Geometry: final body of the model. Coordinates: model frame, mm. A direction names the side the tool comes from. Give positions to 0.01 mm unless a question says otherwise; leave off trailing zeros. Write each loop counter-clockwise with the first axis right and the second up, starting at its lowest first coordinate (ties: lowest second). Pieces come first, ordered by that corner, then holes. Notation, with made-up numbers: (33, -34.75) -> (62, -34.75) arc R30 cw to (62, -4.75) -> close; hole circle Ø1 at (29, 57). An arc over 180 degrees is marked (long way). Answer as a JSON object with one key per item and string values. Group by question number.
(1) Material intervals for probe 1 along Z at (x, y) = (179.5, 129) (3 decimals); probe 2 along Y at (x, z) = (51.5, -41.5) (3 decimals); probe 3 along Y at (x, z) = (146, -30.5) (3 decimals), sorted ascending.
(2) Section query A-A on z = -16.5. Output: boundary loops of the cut face in (x, y) (3 decimals).
(3) Draft query along Y for faces 1 (the face through (273.05, 3, -22)), 2 (the face through (138.44, 1.86, -1.76)), 3 (the face through (118.793, 123.69, -1.565)). Return one class per face: +Y half, -Y half, draft (parallel to the pull), parting line (faces both ways), or undercut.
(4) Contact query for flat-ended pins moving along their axis: pin 1 Ø12 at (y, z) = (167.5, -31.5) entering from -X; pin 2 Ø4 at (x, z) = (160, -29.5) entering from +Y; pin 3 Ø1.6 at (y, z) = (100, -1.5) entering from +X. Output: stop coordinate, or through.
(5) Set-up query: faces 4 (the face through (276.18, 30.21, -1.57)), 5 (the face through (166.5, 64.62, -1.61)), 6 (the face through (149.613, 168.955, -19.142)). Return all of +Z, -Z, +X, -X, +Y, -Y with unobstructed straight access to the full face (end or side cutting, diameter ignored); none if empty.
from build123d import *

# Parameters (mm, degrees)
BASE_FLANGE1_DEPTH           = 3.175
EDGE_FLANGE1_DEPTH           = 350.229988722
EDGE_FLANGE2_STRIP_W         = 18.7
EDGE_FLANGE2_STRIP_H         = 3.175
EDGE_FLANGE2_STRIP_CUT_DEPTH = 273.05
EDGE_FLANGE2_DEPTH           = 273.05
CUT_EXTRUDE1_DEPTH           = 408.732521351
FILLET1_R                    = 12.7
F_11_0_191_DIAMETER_HOLE1_D  = 4.8514
BOSS_EXTRUDE1_DEPTH          = 3.175
FILLET2_R                    = 6.35


# Sheet-metal steps are written as plain solids
with BuildPart() as part:
    # Sketch1 → Base-Flange1 (new body)
    with BuildSketch(Plane.XY):
        Polygon((0, 0), (273.05, 0), (273.05, 41.275), (25.4, 288.925), (0, 288.925), align=None)
    extrude(amount=-BASE_FLANGE1_DEPTH)

    # Edge-Flange1 section (across the edge) → Edge-Flange1 (add)
    with BuildSketch(Plane(origin=(27.521320344, 291.046320344, -3.175), x_dir=(-0.7071067811865436, -0.7071067811865516, -3.4914813388431334e-15), z_dir=(0.7071067811865516, -0.7071067811865436, 0))):
        with BuildLine():
            Line((-3.175, 3), (-3.175, 28.575))
            Line((-3.175, 28.575), (0, 28.575))
            Line((0, 28.575), (0, 3))
            ThreePointArc((0, 3), (0.878679656, 0.878679656), (3, 0))
            Line((3, 0), (3, -3.175))
            ThreePointArc((3, -3.175), (-1.366384374, -1.366384374), (-3.175, 3))
        make_face()
    extrude(amount=EDGE_FLANGE1_DEPTH)

    # Edge-Flange2 strip (across the edge) → Edge-Flange2 strip cut (cut)
    with BuildSketch(Plane(origin=(273.05, 0, -3.175), x_dir=(0, 1, 0), z_dir=(-1, 0, 0))):
        with Locations((-3.175, -1.5875)):
            Rectangle(EDGE_FLANGE2_STRIP_W, EDGE_FLANGE2_STRIP_H)
    extrude(amount=EDGE_FLANGE2_STRIP_CUT_DEPTH, mode=Mode.SUBTRACT)

    # Edge-Flange2 section (across the edge) → Edge-Flange2 (add)
    with BuildSketch(Plane(origin=(273.05, 0, -3.175), x_dir=(0, 1, 0), z_dir=(-1, 0, 0))):
        with BuildLine():
            Line((0, 3), (0, 53.975))
            Line((0, 53.975), (3.175, 53.975))
            Line((3.175, 53.975), (3.175, 3))
            ThreePointArc((3.175, 3), (4.053679656, 0.878679656), (6.175, 0))
            Line((6.175, 0), (6.175, -3.175))
            ThreePointArc((6.175, -3.175), (1.808615626, -1.366384374), (0, 3))
        make_face()
    extrude(amount=EDGE_FLANGE2_DEPTH)

    # Sketch12 → Cut-Extrude1 (cut, through all)
    with BuildSketch(Plane.XY):
        Polygon((50.8, 191.682951031), (50.8, 56.975), (185.507951031, 56.975), align=None)
    extrude(amount=-CUT_EXTRUDE1_DEPTH, mode=Mode.SUBTRACT)

    # Fillet1
    fillet1_edges = [part.edges().sort_by_distance(p)[0] for p in [
        (185.507951031, 56.975, -1.5875),
        (50.8, 56.975, -1.5875),
        (50.8, 191.682951031, -1.5875),
    ]]
    fillet(fillet1_edges, radius=FILLET1_R)

    # #11 (0.191) Diameter Hole1 (through all)
    with Locations(Plane(origin=(0, 0, -3.175), x_dir=(-1, 0, 0), z_dir=(0, 0, -1))):
        with Locations((-22.225, 254), (-22.225, 177.8)):
            Hole(F_11_0_191_DIAMETER_HOLE1_D / 2)

    # Sketch15 → Boss-Extrude1 (add)
    with BuildSketch(Plane.XY):
        Polygon((273.05, 33.3375), (279.4, 26.9875), (279.4, 19.05), (273.05, 12.7), align=None)
    extrude(amount=-BOSS_EXTRUDE1_DEPTH)

    # Fillet2
    fillet2_edges = [part.edges().sort_by_distance(p)[0] for p in [
        (28.643852359, 292.168852359, -31.75),
        (276.293852359, 44.518852359, -31.75),
        (273.05, 1.5875, -57.15),
        (0, 1.5875, -57.15),
        (0, 288.925, -1.5875),
    ]]
    fillet(fillet2_edges, radius=FILLET2_R)


solid = part.part
Answer list:
{
 "1": {"probe 1": "-3.175 to 0", "probe 2": "0 to 3.175", "probe 3": "0 to 3.175, 172.568 to 177.058"},
 "2": {"outline": "(0, 0) -> (273.05, 0) -> (273.05, 3.175) -> (0, 3.175) -> close; (27.521, 291.046) -> (275.171, 43.396) -> (277.416, 45.641) -> (29.766, 293.291) -> close"},
 "3": {"face 1": "draft", "face 2": "-Y half", "face 3": "undercut"},
 "4": {"pin 1": "x = 145.07", "pin 2": "y = 165.06", "pin 3": "x = 221.42"},
 "5": {"face 4": "+Z, -Z, +X", "face 5": "+Z, -Z", "face 6": "-Z, -X"}
}
